Part print with two shaded views. Sizes in mm from the minimum x, y, z corner. Give positions to 0.01 mm unless a question says otherwise; leave off trailing zeros. Write each loop counter-clockwise with the first axis right and the second up, starting at its lowest first coordinate (ties: lowest second). Pieces come first, ordered by that corner, then holes. Notation, with made-up numbers: (48, 76) -> (58, 76) arc R22 ccw to (58, 108) -> close; hole circle Ø10 at (74, 26.5). An arc over 180 degrees is marked (long way). Answer as a JSON object with one key per item and string values.
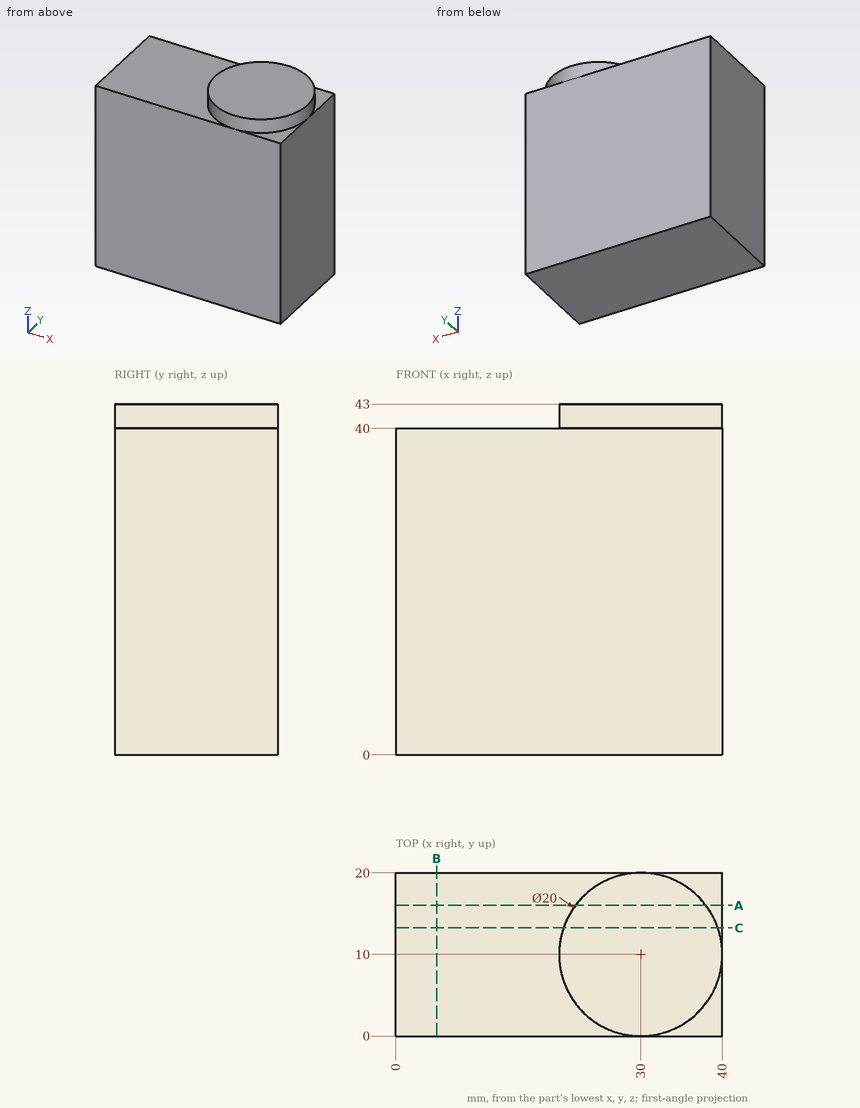
1) Wall check: probe 1 along Z at (x, y) = (17, 11.5). Give the ranges that are in metal, low to high.
Model answer:
{"probe 1": "z = 0 to 40"}
2) Slice it at A-A (y = 16). List the corners of the cut face in (x, z).
Model answer:
{"outline": "(0, 0) -> (40, 0) -> (40, 40) -> (38, 40) -> (38, 43) -> (22, 43) -> (22, 40) -> (0, 40) -> close"}
3) Pin check, flat tip, straight feed: pin 1 (2 mm diameter, centred on x = 7, y = 8, fed in from +Z). Stop position of the tip, or through.
Model answer:
{"pin 1": "stops at z = 40"}
4) Slice it at B-B (x = 5). List the corners of the cut face in (y, z).
Model answer:
{"outline": "(0, 0) -> (20, 0) -> (20, 40) -> (0, 40) -> close"}
5) Slice it at C-C (y = 13.25). List the corners of the cut face in (x, z).
Model answer:
{"outline": "(0, 0) -> (40, 0) -> (40, 40) -> (39.46, 40) -> (39.46, 43) -> (20.54, 43) -> (20.54, 40) -> (0, 40) -> close"}
